Autodesk Fusion 360 part; units mm, degrees
sketch "Boceto1" plane through (0, 0, 0) normal (0, 0, 1) x (1, 0, 0)
  line L0 (96.4, 46.5) -> (-96.4, 46.5)
  line L1 (-96.4, 46.5) -> (-96.4, -46.5)
  line L2 (-96.4, -46.5) -> (96.4, -46.5)
  line L3 (96.4, -46.5) -> (96.4, 46.5)
  line L4 (96.4, 46.5) -> (-96.4, -46.5) construction
  line L5 (-96.4, 46.5) -> (96.4, -46.5) construction
  dimension "d1" = 192.8
  dimension "d2" = 93
extrude "Extruir1" add sketch "Boceto1" along normal blind 56
shell "Vaciado1" thickness 5 removed faces 1 at (-32.1333, 15.5, 56)
fillet "Empalme1" radius 5 1 edges at (96.4, 46.5, 28)
fillet "Empalme2" radius 5 1 edges at (96.4, -46.5, 28)
fillet "Empalme3" radius 5 1 edges at (-96.4, -46.5, 28)
fillet "Empalme4" radius 5 1 edges at (-96.4, 46.5, 28)
sketch "Boceto3" plane through (0, 46.5, 0) normal (0, 1, 0) x (-1, 0, 0)
  line L0 (91.4, 0) -> (91.4, 56)
  line L1 (91.4, 56) -> (-91.4, 56)
  line L2 (-91.4, 56) -> (-91.4, 0)
  line L3 (-91.4, 0) -> (91.4, 0)
  line L4 (-91.4, 0) -> (-91.4, 5)
  line L5 (-91.4, 5) -> (-48.4, 5)
  line L6 (-48.4, 5) -> (-7.4, 5)
  line L7 (-7.4, 5) -> (-7.4, 11)
  line L8 (-7.4, 11) -> (-48.4, 11)
  line L9 (-48.4, 11) -> (-48.4, 5)
  dimension "d17" = 5
  dimension "d18" = 43
  dimension "d19" = 41
  dimension "d20" = 6
  dimension "d21" = 41
extrude "Extruir2" cut sketch "Boceto3" against normal blind 5 contours L6 L7 L8 L9
sketch "Boceto4" plane through (0, 0, 56) normal (0, 0, 1) x (-1, 0, 0)
  arc A0 (91.4, -46.5) -> (96.4, -41.5) centre (91.4, -41.5) ccw
  line L0 (96.4, -41.5) -> (96.4, 41.5)
  arc A1 (96.4, 41.5) -> (91.4, 46.5) centre (91.4, 41.5) ccw
  line L1 (91.4, 46.5) -> (-91.4, 46.5)
  arc A2 (-91.4, 46.5) -> (-96.4, 41.5) centre (-91.4, 41.5) ccw
  line L2 (-96.4, 41.5) -> (-96.4, -41.5)
  arc A3 (-96.4, -41.5) -> (-91.4, -46.5) centre (-91.4, -41.5) ccw
  line L3 (-91.4, -46.5) -> (91.4, -46.5)
  line L4 (-91.4, 41.5) -> (91.4, 41.5)
  line L5 (91.4, 41.5) -> (91.4, -41.5)
  line L6 (91.4, -41.5) -> (-91.4, -41.5)
  line L7 (-91.4, -41.5) -> (-91.4, 41.5)
  line L8 (-96.4, -46.5) -> (-86.4, -46.5)
  line L9 (-86.4, -46.5) -> (-86.4, -44)
  dimension "d24" = 10
  dimension "d25" = 2.5
sketch "Boceto5" plane through (0, 0, 0) normal (0, 0, 1) x (1, 0, 0)
sketch "Boceto6" plane through (0, 0, 56) normal (0, 0, 1) x (-1, 0, 0)
sketch "Boceto7" plane through (0, 0, 56) normal (0, 0, 1) x (-1, 0, 0)
hole "Agujero1" at (86.4, 44, 56) direction (0, 0, -1) diameter 0.769 depth 2 tip angle 118
sketch "Boceto8" plane through (0, 0, 0) normal (0, 0, 1) x (1, 0, 0)
sketch "Boceto9" plane through (0, 0, 56) normal (0, 0, 1) x (-1, 0, 0)
  circle A0 centre (-86.4, -44) radius 0.3847
  arc A1 (91.4, -46.5) -> (96.4, -41.5) centre (91.4, -41.5) ccw
  line L0 (96.4, -41.5) -> (96.4, 41.5)
  arc A2 (96.4, 41.5) -> (91.4, 46.5) centre (91.4, 41.5) ccw
  line L1 (91.4, 46.5) -> (-91.4, 46.5)
  arc A3 (-91.4, 46.5) -> (-96.4, 41.5) centre (-91.4, 41.5) ccw
  line L2 (-96.4, 41.5) -> (-96.4, -41.5)
  arc A4 (-96.4, -41.5) -> (-91.4, -46.5) centre (-91.4, -41.5) ccw
  line L3 (-91.4, -46.5) -> (91.4, -46.5)
  line L4 (-91.4, 41.5) -> (91.4, 41.5)
  line L5 (91.4, 41.5) -> (91.4, -41.5)
  line L6 (91.4, -41.5) -> (-91.4, -41.5)
  line L7 (-91.4, -41.5) -> (-91.4, 41.5)
  line L8 (81.8102, -46.5) -> (81.8102, -44)
  dimension "d31" = 2.5
hole "Agujero2" at (-81.8102, 44, 56) direction (0, 0, -1) diameter 0.769 depth 2 tip angle 118
sketch "Boceto10" plane through (0, 0, 56) normal (0, 0, 1) x (-1, 0, 0)
  circle A0 centre (81.8102, -44) radius 0.3847
  circle A1 centre (-86.4, -44) radius 0.3847
  arc A2 (91.4, -46.5) -> (96.4, -41.5) centre (91.4, -41.5) ccw
  line L0 (96.4, -41.5) -> (96.4, 41.5)
  arc A3 (96.4, 41.5) -> (91.4, 46.5) centre (91.4, 41.5) ccw
  line L1 (91.4, 46.5) -> (-91.4, 46.5)
  arc A4 (-91.4, 46.5) -> (-96.4, 41.5) centre (-91.4, 41.5) ccw
  line L2 (-96.4, 41.5) -> (-96.4, -41.5)
  arc A5 (-96.4, -41.5) -> (-91.4, -46.5) centre (-91.4, -41.5) ccw
  line L3 (-91.4, -46.5) -> (91.4, -46.5)
  line L4 (-91.4, 41.5) -> (91.4, 41.5)
  line L5 (91.4, 41.5) -> (91.4, -41.5)
  line L6 (91.4, -41.5) -> (-91.4, -41.5)
  line L7 (-91.4, -41.5) -> (-91.4, 41.5)
  line L8 (78.4029, 46.5) -> (78.4029, 44)
  line L9 (-85.7578, 46.5) -> (-85.7578, 44)
  dimension "d37" = 2.5
  dimension "d38" = 2.5
hole "Agujero3" at (-78.4029, -44, 56) direction (0, 0, -1) diameter 0.769 depth 2 tip angle 118
sketch "Boceto11" plane through (0, 0, 56) normal (0, 0, 1) x (-1, 0, 0)
  circle A0 centre (78.4029, 44) radius 0.3847
  circle A1 centre (81.8102, -44) radius 0.3847
  circle A2 centre (-86.4, -44) radius 0.3847
  arc A3 (91.4, -46.5) -> (96.4, -41.5) centre (91.4, -41.5) ccw
  line L0 (96.4, -41.5) -> (96.4, 41.5)
  arc A4 (96.4, 41.5) -> (91.4, 46.5) centre (91.4, 41.5) ccw
  line L1 (91.4, 46.5) -> (-91.4, 46.5)
  arc A5 (-91.4, 46.5) -> (-96.4, 41.5) centre (-91.4, 41.5) ccw
  line L2 (-96.4, 41.5) -> (-96.4, -41.5)
  arc A6 (-96.4, -41.5) -> (-91.4, -46.5) centre (-91.4, -41.5) ccw
  line L3 (-91.4, -46.5) -> (91.4, -46.5)
  line L4 (-91.4, 41.5) -> (91.4, 41.5)
  line L5 (91.4, 41.5) -> (91.4, -41.5)
  line L6 (91.4, -41.5) -> (-91.4, -41.5)
  line L7 (-91.4, -41.5) -> (-91.4, 41.5)
  line L8 (-86.4, 46.5) -> (-86.4, 44)
  dimension "d44" = 2.5
hole "Agujero4" at (86.4, -44, 56) direction (0, 0, -1) diameter 0.769 depth 2 tip angle 118
Check sheet for the modelled part. Datum: model origin and axes. Units: mm. A direction names the side the tool comes from. Give positions to 0.01 mm unless a question says otherwise; leave off trailing zeros. Order: outer loops, then holes, each group sorted by start corner. A loop starts at its lowest first (then second) coordinate and runs counter-clockwise, first axis right, second up. Notation, with made-up numbers: M 11.25,51.25 L 56.25,51.25 A12 ccw 56.25,58.25 Z; hole C 83,32 d9. An arc over 180 degrees is marked long. Answer in a Markdown table with one row per item.
1) Cross-section at A-A, the plane z = 26. Enter the section's corners in (x, y), plus the area to 3 significant figures.
Filled sheet:
| item | result |
|---|---|
| outline | M -96.4,-41.5 A5 ccw -91.4,-46.5 L 91.4,-46.5 A5 ccw 96.4,-41.5 L 96.4,41.5 A5 ccw 91.4,46.5 L -91.4,46.5 A5 ccw -96.4,41.5 Z; hole M -91.4,-41.5 L 91.4,-41.5 L 91.4,41.5 L -91.4,41.5 Z |
| area | 2,740 mm2 |
2) Cross-section at C-C, the plane y = 32.5. Enter the section's corners in (x, z), plus the area to 3 significant figures.
Filled sheet:
| item | result |
|---|---|
| outline | M -96.4,0 L 96.4,0 L 96.4,56 L 91.4,56 L 91.4,5 L -91.4,5 L -91.4,56 L -96.4,56 Z |
| area | 1,470 mm2 |
3) Cross-section at D-D, the plane x = -8. Enter the section's corners in (y, z), plus the area to 3 significant figures.
Filled sheet:
| item | result |
|---|---|
| outline | M -46.5,0 L 46.5,0 L 46.5,56 L 41.5,56 L 41.5,5 L -41.5,5 L -41.5,56 L -46.5,56 Z |
| area | 975 mm2 |
4) Thickness scan on L1, parallel to Y at x = 86.4, z = 54.7; L2, parallel to Y at x = 14.5, z = 48.5; L3, parallel to X at y = -44, z = 55. Record the ranges inside material, lowest first. Write a range as [from, to].
Filled sheet:
| item | result |
|---|---|
| L1 | y = [-46.5, -44.38], [-43.62, -41.5], [41.5, 43.62], [44.38, 46.5] |
| L2 | y = [-46.5, -41.5], [41.5, 46.5] |
| L3 | x = [-95.73, -78.79], [-78.02, 86.02], [86.78, 95.73] |
5) Release check for a two-part mould opening along Z. For faces 4 (the flat face through (48.4, 44, 8)), 5 (the flat face through (0, 42, 56)), 6 (the flat face through (-1, -46.5, 28)) record: +Z half, -Z half, draft (parallel to the pull), parting line (faces both ways), or undercut.
Filled sheet:
| item | result |
|---|---|
| face 4 | undercut |
| face 5 | +Z half |
| face 6 | draft |
6) Cross-section at B-B, the plane x = 46. Enter the section's corners in (y, z), plus the area to 3 significant figures.
Filled sheet:
| item | result |
|---|---|
| outline | M -46.5,0 L 46.5,0 L 46.5,5 L -41.5,5 L -41.5,56 L -46.5,56 Z; M 41.5,11 L 46.5,11 L 46.5,56 L 41.5,56 Z |
| area | 945 mm2 |
7) Gauge pin test, flat ends, axial feed: P1, Ø2.5, axis at y = 45, z = 7.5, coming from the -X side; P2, Ø10, axis at x = 61, y = 19.5, coming from the +Z side; P3, Ø1.5, axis at y = 44.5, z = 6.5, coming from the +X side. Record the tip position at first contact, or that the pin passes through.
Filled sheet:
| item | result |
|---|---|
| P1 | stops at x = -95.87 |
| P2 | stops at z = 5 |
| P3 | stops at x = 95.87 |
8) Access from +Z, -Z, +X, -X, +Y, -Y to the whole of each face (thin tool, end or side, straight path). Record for faces 1 (the cylindrical face through (-94.97, -45, 28.39)), 2 (the flat face through (7.4, 44, 8)), 3 (the flat face through (-1, -41.5, 30)).
Filled sheet:
| item | result |
|---|---|
| face 1 | +Z, -Z, -X, -Y |
| face 2 | +Y |
| face 3 | +Z |
